Check sheet for the modelled part. Datum: model origin and axes. Units: mm. Give positions to 0.01 mm unless a question says otherwise; leave off trailing zeros. Loops run counter-clockwise (first coordinate to the right, second up) from the corner with the lowest first, then second, coordinate; pieces in that order, holes last. Notation, with made-up numbers: (66.25, -10) - (92.25, -10) arc R24 ccw to (92.25, 16) - close; hole circle Ø5 at (15, 31). An arc over 180 degrees is marked (long way). Answer in a Markdown table with one row per item. Add a question column.
(1) Sectioned sample at A-A on z = 1.3. Enter the section's corners in (x, y).
(2) Thickness scan on L1, parallel to X at y = 8.5, z = 4; L2, parallel to X at y = 8.75, z = 1.5; L3, parallel to Y at x = 13.25, z = 2.1. Record the ranges inside material, lowest first.
(3) Sectioned sample at D-D on y = -1. Enter the section's corners in (x, z).
(4) Go/stop test with flat-tipped pins: P1, Ø1, axis at y = -1, z = 2.5, coming from the -X side; P2, Ø3, axis at x = 0.5, y = 4.5, coming from the -Z side. Record where each tip stops, or that it passes through.
(5) Sectioned sample at C-C on x = -4.25. Enter the section's corners in (y, z) (3 decimals).
(6) Sectioned sample at B-B on y = 4.25. Enter the section's corners in (x, z).
from build123d import *

# Parameters (mm, degrees)
BOSS_EXTRUDE1_DEPTH = 5


with BuildPart() as part:
    # Sketch1 → Boss-Extrude1 (new body)
    with BuildSketch(Plane.XY):
        with BuildLine():
            ThreePointArc((-12.983067388, 6.118559097), (-11.710745891, 7.734822311), (-10.577139347, 9.451226975))
            ThreePointArc((-10.577139347, 9.451226975), (-9.313293399, 8.406652262), (-7.983008658, 7.448119311))
            ThreePointArc((-7.983008658, 7.448119311), (-3.828474377, 5.202168871), (0.677245379, 3.78691697))
            ThreePointArc((0.677245379, 3.78691697), (5.182965136, 5.202168871), (9.337499417, 7.448119311))
            ThreePointArc((9.337499417, 7.448119311), (10.667784158, 8.406652262), (11.931630106, 9.451226975))
            ThreePointArc((11.931630106, 9.451226975), (13.065236649, 7.734822311), (14.337558146, 6.118559097))
            ThreePointArc((14.337558146, 6.118559097), (12.119892503, 2.841112967), (9.337499417, 0.027221931))
            ThreePointArc((9.337499417, 0.027221931), (5.25986118, -2.66939146), (0.677245379, -4.37188663))
            ThreePointArc((0.677245379, -4.37188663), (-3.905370421, -2.66939146), (-7.983008658, 0.027221931))
            ThreePointArc((-7.983008658, 0.027221931), (-10.765401744, 2.841112967), (-12.983067388, 6.118559097))
        make_face()
    extrude(amount=BOSS_EXTRUDE1_DEPTH)


solid = part.part
Reply:
| question | item | result |
|---|---|---|
| 1 | outline | (-12.98, 6.12) arc R21.43 ccw to (0.68, -4.37) arc R21.43 ccw to (14.34, 6.12) arc R24.73 cw to (11.93, 9.45) arc R24.73 cw to (0.68, 3.79) arc R24.73 cw to (-10.58, 9.45) arc R24.73 cw to start |
| 2 | L1 | -11.18 to -9.43, 10.79 to 12.53 |
| 2 | L2 | -11.02 to -9.75, 11.1 to 12.37 |
| 2 | L3 | 4.35 to 7.48 |
| 3 | outline | (-6.66, 0) - (8.01, 0) - (8.01, 5) - (-6.66, 5) - close |
| 4 | P1 | x = -7.33 |
| 4 | P2 | z = 0 |
| 5 | outline | (-2.49, 0) - (5.385, 0) - (5.385, 5) - (-2.49, 5) - close |
| 6 | outline | (-11.83, 0) - (-1.16, 0) - (-1.16, 5) - (-11.83, 5) - close; (2.51, 0) - (13.18, 0) - (13.18, 5) - (2.51, 5) - close |
